Verification items for the finished model (mm, model axes). Face numbers are marked on the shaded views. A direction names the side the tool comes from. Coordinates: 2 decimals unless noted, no trailing zeros. Order: outer loops, then holes, each group sorted by start corner. A loop starts at its lowest first (then second) coordinate and runs counter-clockwise, first axis right, second up. Notation, with made-up numbers: M 12,15.25 L 65,15.25 A23 ccw 65,23.25 Z; hole C -28.5,9 d7. An arc over 180 degrees is marked long. Return JSON: item names as keys, results as strings. Group by question number.
Q1. Section check C-C, the plane z = 21.5. Enter the section's corners in (x, y).
Q2. Thickness scan on probe 1 along Z at (x, y) = (-33, 77); probe 2 along Z at (x, y) = (15.5, 41); probe 3 along X at (y, z) = (-66.5, 37). Record the ranges inside material, lowest first.
Q3. Section check B-B, the plane y = -20. Enter the section's corners in (x, z).
Q4. Section check A-A, the plane x = 36. Enter the section's corners in (y, z), then the cut area to 3 significant figures.
Q5. Mould release check, pull along Z, two halves, no side actions. Record for the marked faces 1, 2 and 3: pulls with the +Z half, pulls with the -Z half, needs draft (parallel to the pull), parting line crosses it, or undercut.
Q6. Access from +Z, -Z, +X, -X, +Y, -Y to the whole of each face (thin tool, end or side, straight path). Record for the marked faces 4, 5, 6 and 7.
Q7. Go/stop test with flat-tipped pins: pin 1 Ø4.5 at (x, z) = (40, 23) entering from +Y; pin 2 Ø24 at (y, z) = (-72.5, 30) entering from -X; pin 3 Ø1.5 at (x, y) = (31, -47.5) entering from +Z; pin 4 Ø12 at (x, z) = (-2, 0) entering from -Y. Record where each tip stops, or that it passes through.
Q8. Section check D-D, the plane x = 15.5. Enter the section's corners in (y, z).
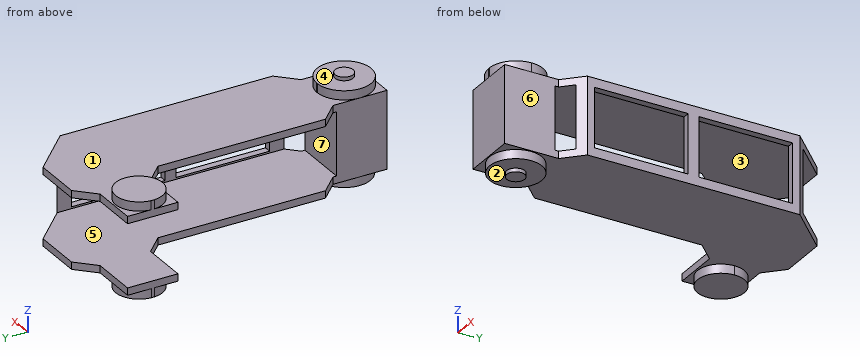
from build123d import *

# Parameters (mm, degrees)
SKETCH1_R           = 14.5
BOSS_EXTRUDE1_DEPTH = 43
SKETCH1_5_R         = 14.5
BOSS_EXTRUDE2_DEPTH = 43
BOSS_EXTRUDE3_DEPTH = 43
BOSS_EXTRUDE4_DEPTH = 5
SKETCH1_8_R         = 14.5
BOSS_EXTRUDE5_DEPTH = 5
SKETCH3_R           = 5
BOSS_EXTRUDE6_DEPTH = 2
BOSS_EXTRUDE7_DEPTH = 5
BOSS_EXTRUDE8_DEPTH = 5
SKETCH5_R           = 5
BOSS_EXTRUDE9_DEPTH = 2
SKETCH6_W           = 17.5
SKETCH6_H           = 27.979977464
CUT_EXTRUDE1_DEPTH  = 82
SKETCH7_W           = 19.05
SKETCH7_H           = 35
SKETCH7_W_2         = 13.5
CUT_EXTRUDE4_DEPTH  = 153
SKETCH9_W           = 33
SKETCH9_H           = 52
CUT_EXTRUDE5_DEPTH  = 33


with BuildPart() as part:
    # Sketch1 → Boss-Extrude1 (new body)
    with BuildSketch(Plane.XY):
        with BuildLine():
            Line((-17, 80.5), (-42.944942798, 80.5))
            Line((-42.944942798, 80.5), (-42.944942798, 67.345568333))
            ThreePointArc((-42.944942798, 67.345568333), (-29.549463234, 79.493116027), (-16.972471399, 66.5))
            ThreePointArc((-16.972471399, 66.5), (-29.549463234, 53.506883973), (-42.944942798, 65.654431667))
            Line((-42.944942798, 65.654431667), (-42.944942798, 52.520022536))
            Line((-42.944942798, 52.520022536), (-17, 52.520022536))
            Line((-17, 52.520022536), (-7, 42.520022536))
            Line((-7, 42.520022536), (-7, -50.479977464))
            Line((-7, -50.479977464), (3, -60.479977464))
            Line((3, -60.479977464), (3, -90.479977464))
            Line((3, -90.479977464), (33, -90.479977464))
            Line((33, -90.479977464), (33, -60.5))
            Line((33, -60.5), (43, -50.5))
            Line((43, -50.5), (43, 67.5))
            Line((43, 67.5), (20, 90.5))
            Line((20, 90.5), (-7, 90.5))
            Line((-7, 90.5), (-17, 80.5))
        make_face()
        with Locations((17.898375843, -75.5)):
            Circle(SKETCH1_R, mode=Mode.SUBTRACT)
    extrude(amount=BOSS_EXTRUDE1_DEPTH)

    # Sketch1_5 → Boss-Extrude2 (add)
    with BuildSketch(Plane.XY):
        with Locations((17.898375843, -75.5)):
            Circle(SKETCH1_5_R)
    extrude(amount=BOSS_EXTRUDE2_DEPTH)

    # Sketch1_6 → Boss-Extrude3 (add)
    with BuildSketch(Plane.XY):
        with BuildLine():
            ThreePointArc((-16.972471399, 66.5), (-29.549463234, 79.493116027), (-42.944942798, 67.345568333))
            Line((-42.944942798, 67.345568333), (-42.944942798, 65.654431667))
            ThreePointArc((-42.944942798, 65.654431667), (-29.549463234, 53.506883973), (-16.972471399, 66.5))
        make_face()
    extrude(amount=BOSS_EXTRUDE3_DEPTH)

    # Sketch1_7 → Boss-Extrude4 (add)
    with BuildSketch(Plane.XY):
        with BuildLine():
            ThreePointArc((-16.972471399, 66.5), (-29.549463234, 79.493116027), (-42.944942798, 67.345568333))
            Line((-42.944942798, 67.345568333), (-42.944942798, 65.654431667))
            ThreePointArc((-42.944942798, 65.654431667), (-29.549463234, 53.506883973), (-16.972471399, 66.5))
        make_face()
    extrude(amount=-BOSS_EXTRUDE4_DEPTH)

    # Sketch1_8 → Boss-Extrude5 (add)
    with BuildSketch(Plane.XY):
        with Locations((17.898375843, -75.5)):
            Circle(SKETCH1_8_R)
    extrude(amount=-BOSS_EXTRUDE5_DEPTH)

    # Sketch3 → Boss-Extrude6 (add)
    with BuildSketch(Plane(origin=(0, 0, -5), x_dir=(-1, 0, 0), z_dir=(0, 0, -1))):
        with Locations((-17.898375843, -75.5)):
            Circle(SKETCH3_R)
    extrude(amount=BOSS_EXTRUDE6_DEPTH)

    # Sketch4 → Boss-Extrude7 (add)
    with BuildSketch(Plane.XY.offset(43)):
        with BuildLine():
            Line((-17, 66.510011268), (-17, 67.355579601))
            ThreePointArc((-17, 67.355579601), (-29.972471399, 79.510011268), (-42.944942798, 67.355579601))
            Line((-42.944942798, 67.355579601), (-42.944942798, 66.510011268))
            Line((-42.944942798, 66.510011268), (-17, 66.510011268))
        make_face()
        with BuildLine():
            Line((-17, 65.664442935), (-17, 66.510011268))
            Line((-17, 66.510011268), (-42.944942798, 66.510011268))
            Line((-42.944942798, 66.510011268), (-42.944942798, 65.664442935))
            ThreePointArc((-42.944942798, 65.664442935), (-29.972471399, 53.510011268), (-17, 65.664442935))
        make_face()
    extrude(amount=BOSS_EXTRUDE7_DEPTH)

    # Sketch4_3 → Boss-Extrude8 (add)
    with BuildSketch(Plane.XY.offset(43)):
        with BuildLine():
            Line((18, -60.489988732), (17.62239464, -60.489736711))
            ThreePointArc((17.62239464, -60.489736711), (3.000000814, -75.480042097), (17.612515852, -90.479977464))
            Line((17.612515852, -90.479977464), (18, -90.479977464))
            Line((18, -90.479977464), (18, -60.489988732))
        make_face()
        with BuildLine():
            Line((18.397621205, -60.490254111), (18, -60.489988732))
            Line((18, -60.489988732), (18, -90.479977464))
            Line((18, -90.479977464), (18.387484148, -90.479977464))
            ThreePointArc((18.387484148, -90.479977464), (28.742724566, -85.953692134), (33, -75.484983098))
            ThreePointArc((33, -75.484983098), (28.746262561, -65.01990589), (18.397621205, -60.490254111))
        make_face()
    extrude(amount=BOSS_EXTRUDE8_DEPTH)

    # Sketch5 → Boss-Extrude9 (add)
    with BuildSketch(Plane.XY.offset(48)):
        with Locations((18, -75.484983098)):
            Circle(SKETCH5_R)
    extrude(amount=BOSS_EXTRUDE9_DEPTH)

    # Sketch6 → Cut-Extrude1 (cut)
    with BuildSketch(Plane.ZY.offset(42.944942798)):
        with Locations((12.75, 66.510011268)):
            Rectangle(SKETCH6_W, SKETCH6_H)
        with Locations((30.25, 66.510011268)):
            Rectangle(SKETCH6_W, SKETCH6_H)
    extrude(amount=-CUT_EXTRUDE1_DEPTH, mode=Mode.SUBTRACT)

    # Sketch7 → Cut-Extrude4 (cut)
    with BuildSketch(Plane(origin=(0, 90.5, 0), x_dir=(1, 0, 0), z_dir=(0, 1, 0))):
        with Locations((-16.525, -21.5)):
            Rectangle(SKETCH7_W, SKETCH7_H)
        with Locations((-0.25, -21.5)):
            Rectangle(SKETCH7_W_2, SKETCH7_H)
        with Locations((13.25, -21.5)):
            Rectangle(SKETCH7_W_2, SKETCH7_H)
        with Locations((29.525, -21.5)):
            Rectangle(SKETCH7_W, SKETCH7_H)
    extrude(amount=-CUT_EXTRUDE4_DEPTH, mode=Mode.SUBTRACT)

    # Sketch9 → Cut-Extrude5 (cut)
    with BuildSketch(Plane(origin=(43, 0, 0), x_dir=(0, 0, -1), z_dir=(1, 0, 0))):
        with Locations((-21.5, 37.5)):
            Rectangle(SKETCH9_W, SKETCH9_H)
        with Locations((-21.5, -20.5)):
            Rectangle(SKETCH9_W, SKETCH9_H)
    extrude(amount=-CUT_EXTRUDE5_DEPTH, mode=Mode.SUBTRACT)


solid = part.part
Numbers:
{
 "1": {"outline": "M 3,-90.48 L 33,-90.48 L 33,-62.5 L 3,-62.5 Z; M 39.05,-54.45 L 43,-50.5 L 43,-46.5 L 39.05,-46.5 Z; M 39.05,5.5 L 43,5.5 L 43,11.5 L 39.05,11.5 Z; M 39.06,63.5 L 43,63.5 L 43,67.5 L 39.06,71.44 Z"},
 "2": {"probe 1": "z = -5 to 4, 39 to 48", "probe 2": "z = 0 to 4, 39 to 43", "probe 3": "x = 3 to 33"},
 "3": {"outline": "M -7,0 L 43,0 L 43,5 L 39.05,5 L 39.05,4 L -7,4 Z; M -7,39 L 39.05,39 L 39.05,38 L 43,38 L 43,43 L -7,43 Z"},
 "4": {"outline": "M -57.5,0 L 74.5,0 L 74.5,4 L -57.5,4 Z; M -57.5,39 L 74.5,39 L 74.5,43 L -57.5,43 Z", "area": "1,060 mm2"},
 "5": {"face 1": "pulls with the +Z half", "face 2": "pulls with the -Z half", "face 3": "undercut"},
 "6": {"face 4": "+Z", "face 5": "-X, +Y", "face 6": "+Z, -Z, +X, -Y", "face 7": "+X, -X, +Y"},
 "7": {"pin 1": "stops at y = 71.44", "pin 2": "stops at x = 3", "pin 3": "stops at z = 43", "pin 4": "stops at y = -90.48"},
 "8": {"outline": "M -90.48,0 L -89.8,0 L -89.8,-5 L -79.89,-5 L -79.89,-7 L -71.11,-7 L -71.11,-5 L -61.2,-5 L -61.2,0 L 90.5,0 L 90.5,4 L -62.5,4 L -62.5,39 L 90.5,39 L 90.5,43 L -60.69,43 L -60.69,48 L -71.15,48 L -71.15,50 L -79.82,50 L -79.82,48 L -90.28,48 L -90.28,43 L -90.48,43 Z"}
}
